Answer from the drawing. Dimensions are ordinates in mm from the lowest x, y and z of the part. A direction names the side the tool comes from. Round coordinates to 2 decimals unless told otherwise and drop trailing zeros. Write each loop counter-clockwise with the first axis right and the second up, starting at its lowest first coordinate (ties: lowest second). Pieces come first, ordered by that corner, then holes. Notation, with made-up numbers: (-4.75, -24.5) - (42.25, -24.5) arc R20 ccw to (42.25, -8.5) - close; hole circle Ø7 at (-29.5, -16). An arc over 180 degrees is marked (long way). Answer in a Markdown table with one row per item.
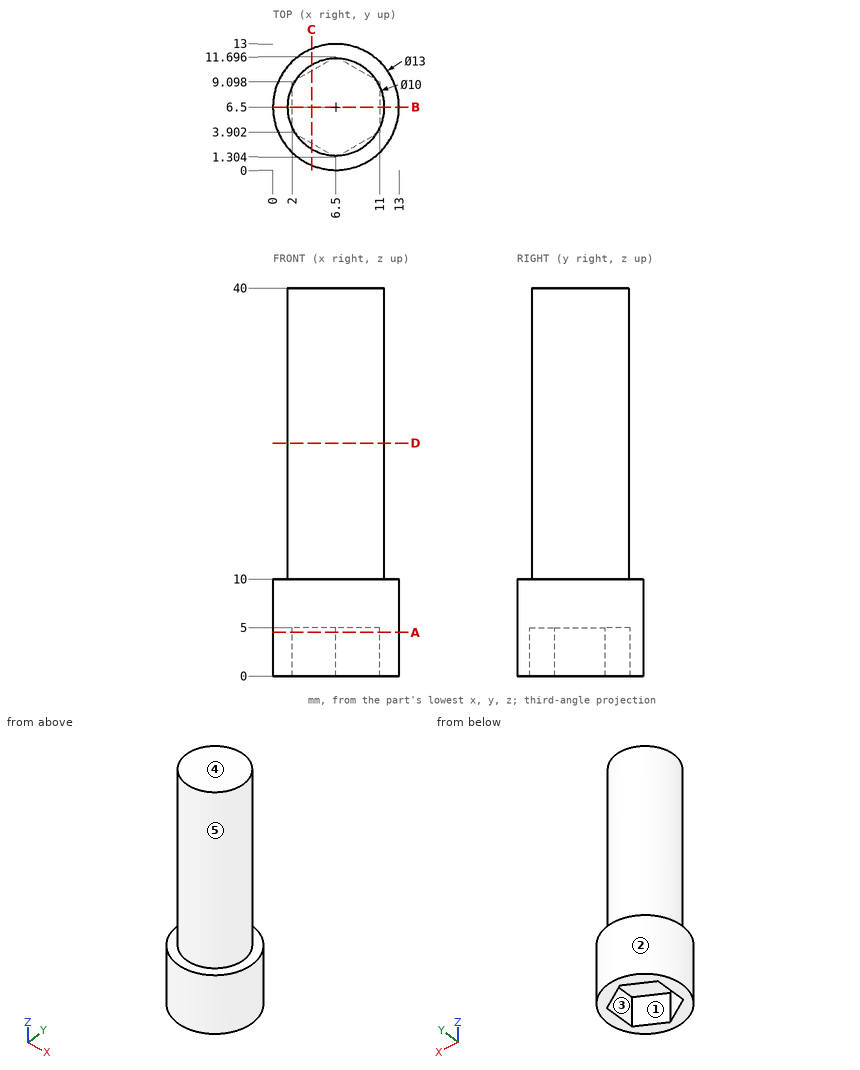
(1) For the marked faces 1 and 2, determine the directions among +Z, -Z, +X, -X, +Y, -Y from which every point of the face is accessible in a straight line to the end or side of a thin tool.
Checked values:
| item | result |
|---|---|
| face 1 | -Z |
| face 2 | +Z, -Z |
(2) Section B-B (y = 6.5) is taken. Give the vertices of the cut face in (x, z).
Checked values:
| item | result |
|---|---|
| outline | (0, 0) - (2, 0) - (2, 5) - (11, 5) - (11, 0) - (13, 0) - (13, 10) - (11.5, 10) - (11.5, 40) - (1.5, 40) - (1.5, 10) - (0, 10) - close |
(3) For a pull along X with two mould halves and no side action, classify the marked faces 3, 4 and 5 as pulls with the +X half, pulls with the -X half, needs draft (parallel to the pull), parting line crosses it, or undercut.
Checked values:
| item | result |
|---|---|
| face 3 | undercut |
| face 4 | needs draft |
| face 5 | parting line crosses it |
(4) Find the intervals of material crossed by line 1 (Z direction, x = 7.75, y = 10.5); line 2 (Z direction, x = 1.5, y = 7.5); line 3 (X direction, y = 6.75, z = 30), in increasing order.
Checked values:
| item | result |
|---|---|
| line 1 | z = 5 to 40 |
| line 2 | z = 0 to 10 |
| line 3 | x = 1.51 to 11.49 |
(5) Section C-C (x = 4) is taken. Give the vertices of the cut face in (y, z), and give its area (3 significant figures).
Checked values:
| item | result |
|---|---|
| outline | (0.5, 0) - (2.75, 0) - (2.75, 5) - (10.25, 5) - (10.25, 0) - (12.5, 0) - (12.5, 10) - (10.83, 10) - (10.83, 40) - (2.17, 40) - (2.17, 10) - (0.5, 10) - close |
| area | 342 mm2 |
(6) Flat-ended cylindrical pins translate along their axes: pin 1 (2.5 mm diameter, centred on y = 8, z = 1.5, fed in from -X) (3 decimals); pin 2 (4.5 mm diameter, centred on x = 5, y = 6.5, fed in from -Z); pin 3 (5 mm diameter, centred on y = 11.5, z = 27.5, fed in from +X). Find the tip coordinate at first contact, or state that the pin passes through.
Checked values:
| item | result |
|---|---|
| pin 1 | stops at x = 0.005 |
| pin 2 | stops at z = 5 |
| pin 3 | stops at x = 10.83 |
(7) Section D-D (z = 24) is taken. Give the vertices of the cut face in (x, y).
Checked values:
| item | result |
|---|---|
| outline | circle Ø10 at (6.5, 6.5) |
(8) Section A-A (z = 4.5) is taken. Give the vertices of the cut face in (x, y).
Checked values:
| item | result |
|---|---|
| outline | circle Ø13 at (6.5, 6.5); hole (2, 3.9) - (6.5, 1.3) - (11, 3.9) - (11, 9.1) - (6.5, 11.7) - (2, 9.1) - close |
